Build history of the part. All positions in model axes, mm. Give positions to 0.01 mm unless a question says otherwise; leave off trailing zeros. Answer in a Markdown table with one row per item.
```python
from build123d import *

# Parameters (mm, degrees)
SKICA1_W                 = 280
SKICA1_H                 = 460
P_IDAT_VYSUNUT_M1_DEPTH  = 10
SKICA3_R                 = 1.75
SKICA3_R_2               = 2.25
ODEBRAT_VYSUNUT_M1_DEPTH = 10
SKICA4_R                 = 1.25
ODEBRAT_VYSUNUT_M2_DEPTH = 10
ZAOBLIT1_R               = 10
ZKOSEN_1_SIZE            = 5


with BuildPart() as part:
    # Skica1 → Přidat vysunutím1 (new body)
    with BuildSketch(Plane.XY):
        with Locations((6, 4.9692)):
            Rectangle(SKICA1_W, SKICA1_H)
    extrude(amount=P_IDAT_VYSUNUT_M1_DEPTH)

    # Skica3 → Odebrat vysunutím1 (cut)
    with BuildSketch(Plane.XY.offset(10)):
        with Locations((25, 135)):
            Circle(SKICA3_R)
        with Locations((25, 105)):
            Circle(SKICA3_R)
        with Locations((-25, 135)):
            Circle(SKICA3_R)
        with Locations((-25, 105)):
            Circle(SKICA3_R)
        with Locations((-102.8, -5.1992)):
            Circle(SKICA3_R_2)
        with Locations((110.186658443, -152.108914912)):
            Circle(SKICA3_R)
        with Locations((110.204187307, -136.108924514)):
            Circle(SKICA3_R)
        with Locations((70.309542186, -152.214237593)):
            Circle(SKICA3_R)
        with Locations((70.207496415, -136.214563013)):
            Circle(SKICA3_R)
        with Locations((114.8, 62.2008)):
            Circle(SKICA3_R_2)
        with Locations((130.2, -5.1992)):
            Circle(SKICA3_R_2)
        with Locations((-118.2, 62.2008)):
            Circle(SKICA3_R_2)
        with Locations((25, -5)):
            Circle(SKICA3_R)
        with Locations((25, -35)):
            Circle(SKICA3_R)
        with Locations((-25, -35)):
            Circle(SKICA3_R)
        with Locations((-25, -5)):
            Circle(SKICA3_R)
    extrude(amount=-ODEBRAT_VYSUNUT_M1_DEPTH, mode=Mode.SUBTRACT)

    # Skica4 → Odebrat vysunutím2 (cut)
    with BuildSketch(Plane.XY.offset(10)):
        with Locations((126, 144.9692)):
            Circle(SKICA4_R)
        with Locations((126, -205.0308)):
            Circle(SKICA4_R)
        with Locations((-114, -205.0308)):
            Circle(SKICA4_R)
        with Locations((-114, 144.9692)):
            Circle(SKICA4_R)
    extrude(amount=-ODEBRAT_VYSUNUT_M2_DEPTH, mode=Mode.SUBTRACT)

    # Zaoblit1
    zaoblit1_edges = [part.edges().sort_by_distance(p)[0] for p in [
        (146, -225.0308, 5),
        (-134, -225.0308, 5),
        (-134, 234.9692, 5),
        (146, 234.9692, 5),
    ]]
    fillet(zaoblit1_edges, radius=ZAOBLIT1_R)

    # Zkosení1
    zkosen_1_edges = [part.edges().sort_by_distance(p)[0] for p in [
        (6, -225.0308, 0),
        (146, 4.9692, 0),
        (-134, 4.9692, 0),
        (6, 234.9692, 0),
        (143.071067812, -222.101867812, 0),
        (143.071067812, 232.040267812, 0),
        (-131.071067812, 232.040267812, 0),
        (-131.071067812, -222.101867812, 0),
    ]]
    chamfer(zkosen_1_edges, length=ZKOSEN_1_SIZE)


solid = part.part
```
1. Probe line 1 (Y direction, x = 126, z = 6); line 2 (Y direction, x = 114.8, z = 5); line 3 (Y direction, x = -118.5, z = 9). List the from-to ranges inside material, lowest first.
Check result:
| item | result |
|---|---|
| line 1 | y = -225.03 to -206.28, -203.78 to 143.72, 146.22 to 234.97 |
| line 2 | y = -225.03 to 59.95, 64.45 to 234.97 |
| line 3 | y = -225.03 to 59.97, 64.43 to 234.97 |
2. Cut at A-A on z = 1.75. Count the separate pieces of the cut face and the enclosed holes in it, and give its area (3 significant figures).
Check result:
| item | result |
|---|---|
| separate pieces | 1 |
| enclosed holes | 20 |
| area | 124,000 mm² |
3. Drop flat-ended pins along their axis: P1, Ø3, axis at x = 110.19, y = -152.11, coming from the +Z side; P2, Ø2, axis at x = 8, z = 2, coming from the -Y side; P3, Ø1.5, axis at x = -102, z = 4, coming from the +Y side; P4, Ø2, axis at x = 5.5, z = 3.5, coming from the +Y side. Give the stop position or say it passes through.
Check result:
| item | result |
|---|---|
| P1 | passes through |
| P2 | stops at y = -223.03 |
| P3 | stops at y = 234.72 |
| P4 | stops at y = 234.47 |
